Can you work these out from the model? Positions are in its coordinate system, mm. Face numbers are marked on the shaded views. A direction names the side the tool comes from. Coordinates: 2 decimals unless noted, no trailing zeros. Loops run counter-clockwise (first coordinate to the right, second up) from the corner with the lowest first, then second, coordinate; pieces in that order, holes last. Notation, with made-up numbers: (84, -23.75) -> (137, -23.75) arc R29 cw to (137, 6.25) -> close; hole circle Ø3 at (35.5, 89). An arc over 180 degrees is marked (long way). Use one line per item in the form item = value. Start each with the question number.
(1) Thinking about a two-plate mould opening in Y: for the marked faces 3, 4 and 5, which applies, released by +Y, released by -Y, zero draft, split by the parting line, or undercut?
(2) Imagine slicing it at A-A (x = 71). List the corners of the cut face in (y, z) for me.
(3) Imagine slicing it at B-B (y = 82). List the corners of the cut face in (x, z) for me, plus the area to 3 significant figures.
(4) Imagine slicing it at C-C (y = 43). List the corners of the cut face in (x, z) for me, plus the area to 3 significant figures.
(5) I'm going to push flat-ended pins straight in: pin 1 (14.5 mm diameter, centred on x = 81, y = 41.5, fed in from +Z); pin 2 (3 mm diameter, centred on x = 135, y = 78, fed in from +Z); pin 3 (8 mm diameter, centred on x = 122, y = 87.5, fed in from +Z). Where does each tip first touch, or does it pass through?
(6) On a 3-axis mill with a long thin cutter (end or side, diameter ignored), from which of +Z, -Z, +X, -X, +Y, -Y can I reach the whole of each face in a straight line? I mean the marked faces 1 and 2. Say none if no direction works.
(7) I need wall thicknesses on line 1 (Y direction, x = 145, z = 30.5); line 2 (Y direction, x = 54, z = 33); line 3 (Z direction, x = 191.5, y = 39). Which ranges of each line are inside material? Lowest first, please. Write a range as [from, to].
```python
from build123d import *

# Parameters (mm, degrees)
SALIENTE_EXTRUIR1_DEPTH = 200


with BuildPart() as part:
    # Croquis1 → Saliente-Extruir1 (new body)
    with BuildSketch(Plane(origin=(0, 0, 0), x_dir=(0, 0, -1), z_dir=(1, 0, 0))):
        with BuildLine():
            Line((0, 0), (-23.183766184, 0))
            ThreePointArc((-23.183766184, 0), (-23.949133049, 0.152240935), (-24.597979746, 0.585786438))
            Line((-24.597979746, 0.585786438), (-37.071067812, 13.058874503))
            ThreePointArc((-37.071067812, 13.058874503), (-39.238795325, 23.956776639), (-30, 30.129942315))
            Line((-30, 30.129942315), (-22, 30.129942315))
            ThreePointArc((-22, 30.129942315), (-20.585786438, 30.715728753), (-20, 32.129942315))
            Line((-20, 32.129942315), (-20, 45.129942315))
            ThreePointArc((-20, 45.129942315), (-20.152240935, 45.89530918), (-20.585786438, 46.544155877))
            Line((-20.585786438, 46.544155877), (-38.535533906, 64.493903346))
            ThreePointArc((-38.535533906, 64.493903346), (-39.619397663, 69.942854413), (-35, 73.029437252))
            Line((-35, 73.029437252), (-32, 73.029437252))
            ThreePointArc((-32, 73.029437252), (-30.585786438, 73.615223689), (-30, 75.029437252))
            Line((-30, 75.029437252), (-30, 85.029437252))
            ThreePointArc((-30, 85.029437252), (-30.152240935, 85.794804116), (-30.585786438, 86.443650814))
            Line((-30.585786438, 86.443650814), (-37.071067812, 92.928932188))
            ThreePointArc((-37.071067812, 92.928932188), (-39.238795325, 103.826834324), (-30, 110))
            Line((-30, 110), (0, 110))
            Line((0, 110), (0, 0))
        make_face()
    extrude(amount=SALIENTE_EXTRUIR1_DEPTH)


solid = part.part
```
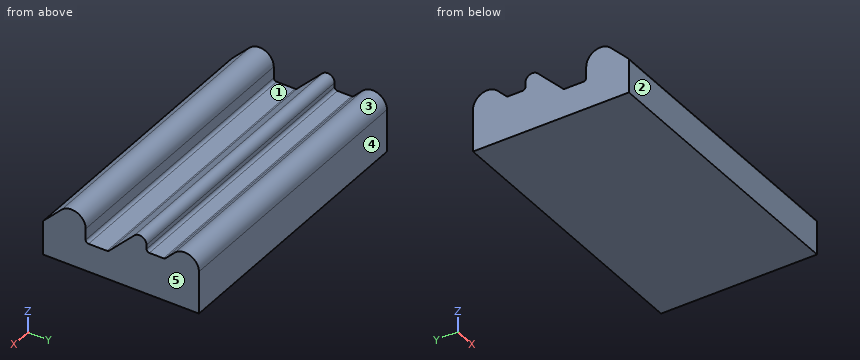
Worked out:
q1.face_3 = undercut
q1.face_4 = released by +Y
q1.face_5 = zero draft
q2.outline = (0, 0) -> (110, 0) -> (110, 30) arc R10 ccw to (92.93, 37.07) -> (86.44, 30.59) arc R2 cw to (85.03, 30) -> (75.03, 30) arc R2 cw to (73.03, 32) -> (73.03, 35) arc R5 ccw to (64.49, 38.54) -> (46.54, 20.59) arc R2 cw to (45.13, 20) -> (32.13, 20) arc R2 cw to (30.13, 22) -> (30.13, 30) arc R10 ccw to (13.06, 37.07) -> (0.59, 24.6) arc R2 ccw to (0, 23.18) -> close
q3.outline = (0, 0) -> (200, 0) -> (200, 30) -> (0, 30) -> close
q3.area = 6,000 mm2
q4.outline = (0, 0) -> (200, 0) -> (200, 20) -> (0, 20) -> close
q4.area = 4,000 mm2
q5.pin_1 = 22.79
q5.pin_2 = 30
q5.pin_3 = 35.64
q6.face_1 = +Z, +X, -X
q6.face_2 = +Z, -Z, +X, -X, -Y
q7.line_1 = [6.49, 30.12], [56.46, 73.71], [86.35, 109.99]
q7.line_2 = [8.99, 29.67], [58.96, 73.03], [88.86, 109.54]
q7.line_3 = [0, 20]
